Verification items for the finished model (mm, model axes). Face numbers are marked on the shaded views. A direction names the side the tool comes from. Round coordinates to 2 decimals unless told otherwise and drop trailing zeros. Write each loop counter-clockwise with the first axis right and the second up, starting at its lowest first coordinate (ties: lowest second). Pieces come first, ordered by that corner, then holes. Notation, with made-up numbers: (57, 71.5) -> (95, 71.5) arc R20 ccw to (95, 106.5) -> close; hole circle Ø4 at (-10.5, 43.25). An arc over 180 degrees is marked (long way). Use CSV: the item, a comma, the result in double quotes.
```python
from build123d import *

# Parameters (mm, degrees)
F1_DEPTH       = 50
F3_D           = 16
F3_CBORE_D     = 30
F3_CBORE_DEPTH = 20
F5_D           = 30
F5_CBORE_D     = 30
F5_CBORE_DEPTH = 20


with BuildPart() as f1:
    # F0 (on Front) → F1 (new body)
    with BuildSketch(Plane.XZ):
        Polygon((0, 100), (-90, 100), (-90, 70), (-15, 70), (-15, -20), (60, -20), (60, 0), (0, 0), align=None)
    extrude(amount=F1_DEPTH)

    # F3 (through all)
    with Locations(Plane.XY.offset(100)):
        with Locations((-60, -25)):
            CounterBoreHole(F3_D / 2, F3_CBORE_D / 2, F3_CBORE_DEPTH)

    # F5 (through all)
    with Locations(Plane.XY):
        with Locations((30, -25)):
            CounterBoreHole(F5_D / 2, F5_CBORE_D / 2, F5_CBORE_DEPTH)


solid = f1.part
```
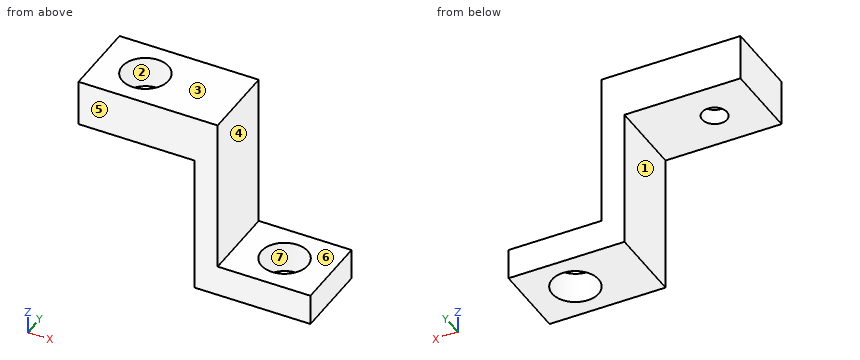
Q1. Section check A-A (x = -60). Record the cut outline in (y, z), plus the area to 3 significant figures.
Filled in:
outline,"(-50, 70) -> (-33, 70) -> (-33, 80) -> (-40, 80) -> (-40, 100) -> (-50, 100) -> close; (-17, 70) -> (0, 70) -> (0, 100) -> (-10, 100) -> (-10, 80) -> (-17, 80) -> close"
area,"740 mm²"
Q2. Go/stop test with flat-tipped pins: P1, Ø3, axis at y = -17.5, z = 53, coming from the +X side; P2, Ø14.5, axis at x = -60, y = -25, coming from the -Z side; P3, Ø18, axis at x = -60, y = -25, coming from the +Z side; P4, Ø4, axis at x = 44, y = -8, coming from the +Z side. Record where each tip stops, or that it passes through.
Filled in:
P1,"x = 0"
P2,"through"
P3,"z = 80"
P4,"z = 0"
Q3. Access from +Z, -Z, +X, -X, +Y, -Y to the whole of each face (thin tool, end or side, straight path). Record for the marked faces 1, 2, 3 and 4.
Filled in:
face 1,"-Z, -X, +Y, -Y"
face 2,"+Z"
face 3,"+Z, +X, -X, +Y, -Y"
face 4,"+Z, +X, +Y, -Y"
Q4. Section check C-C (z = 78). Record the cut outline in (x, y).
Filled in:
outline,"(-90, -50) -> (0, -50) -> (0, 0) -> (-90, 0) -> close; hole circle Ø16 at (-60, -25)"
Q5. Section check D-D (y = -42). Record the cut outline in (x, z).
Filled in:
outline,"(-90, 70) -> (-15, 70) -> (-15, -20) -> (60, -20) -> (60, 0) -> (0, 0) -> (0, 100) -> (-90, 100) -> close"
Q6. Section check B-B (y = -25). Record the cut outline in (x, z), plus the area to 3 significant figures.
Filled in:
outline,"(-90, 70) -> (-68, 70) -> (-68, 80) -> (-75, 80) -> (-75, 100) -> (-90, 100) -> close; (-52, 70) -> (-15, 70) -> (-15, -20) -> (15, -20) -> (15, 0) -> (0, 0) -> (0, 100) -> (-45, 100) -> (-45, 80) -> (-52, 80) -> close; (45, -20) -> (60, -20) -> (60, 0) -> (45, 0) -> close"
area,"3,890 mm²"
Q7. Material ranges on L1, parallel to Y at x = -60, z = 95; L2, parallel to Y at x = -60, z = 76.5; L3, parallel to X at y = -29, z = 27, recorded low to high.
Filled in:
L1,"-50 to -40, -10 to 0"
L2,"-50 to -33, -17 to 0"
L3,"-15 to 0"
Q8. Mould release check, pull along Y, two halves, no side actions. Record for the marked faces 5, 6 and 7: released by +Y, released by -Y, zero draft, split by the parting line, or undercut.
Filled in:
face 5,"released by -Y"
face 6,"zero draft"
face 7,"undercut"
